Autodesk Inventor part; units mm, degrees
ref_plane "YZ Plane" through (0, 0, 0) normal (1, 0, 0) x (0, 1, 0)
ref_plane "XZ Plane" through (0, 0, 0) normal (0, 1, 0) x (-1, 0, 0)
ref_plane "XY Plane" through (0, 0, 0) normal (0, 0, 1) x (1, 0, 0)
sketch "Sketch1" plane through (0, 0, 0) normal (0, 0, 1) x (1, 0, 0)
  circle A0 centre (0, 0) radius 9.75
  dimension "d0" = 19.5
extrude "Extrusion1" add sketch "Sketch1" along normal blind 3
sketch "Sketch2" plane through (0, 0, 0) normal (0, 0, -1) x (-1, 0, 0)
  circle A0 centre (0, 0) radius 7.2
  circle A1 centre (0, 0) radius 4.7
  dimension "d3" = 14.4
  dimension "d4" = 2.5
extrude "Extrusion2" add sketch "Sketch2" along normal blind 6
fillet "Fillet1" radius 2 1 edges at (-9.75, 0, 3)
sketch "Sketch3" plane through (0, 0, 3) normal (0, 0, 1) x (1, 0, 0)
  line L0 (0.8, -4.5) -> (-0.8, -4.5)
  line L1 (-0.8, 4.5) -> (0.8, 4.5)
  line L2 (0.8, -4.5) -> (-0.8, 4.5) construction
  line L3 (-0.8, -4.5) -> (0.8, 4.5) construction
  line L4 (-3, -0.8) -> (-3, 0.8)
  line L5 (3, 0.8) -> (3, -0.8)
  circle A0 centre (0, 0) radius 4.7
  line L6 (3, -0.8) -> (-3, 0.8) construction
  line L7 (-3, -0.8) -> (3, 0.8) construction
  line L8 (3, -0.8) -> (0.8, -0.8)
  line L9 (-0.8, -4.5) -> (-0.8, -0.8)
  line L10 (0.1422, -0.8) -> (-0.1422, -0.8)
  line L11 (-0.8, -0.8) -> (-3, -0.8)
  line L12 (0.8, 0.8) -> (3, 0.8)
  line L13 (-3, 0.8) -> (-0.8, 0.8)
  line L14 (-0.1422, 0.8) -> (0.1422, 0.8)
  line L15 (-0.8, -0.2133) -> (-0.8, 0.2133)
  line L16 (-0.8, 0.8) -> (-0.8, 4.5)
  line L17 (0.8, 4.5) -> (0.8, 0.8)
  line L18 (0.8, 0.2133) -> (0.8, -0.2133)
  line L19 (0.8, -0.8) -> (0.8, -4.5)
  dimension "d8" = 9
  dimension "d9" = 6
extrude "Extrusion3" cut sketch "Sketch3" against normal blind 2 contours L0 L9 L11 L4 L13 L16 L1 L17 L12 L5 L8 L19
thread "Thread1"
chamfer "Chamfer1" distance 1 angle 45 1 edges at (7.2, 0, -6)
equation "\"d11\" = d10"
properties part number "PG9x6mm_Plug"
Here's how the part is built. I have some questions about the finished solid (model axes, mm). A direction names the side the tool comes from. Coordinates: 2 decimals unless noted, no trailing zeros. Loops run counter-clockwise (first coordinate to the right, second up) from the corner with the lowest first, then second, coordinate; pieces in that order, holes last.
1. Imagine slicing it at C-C, the plane y = 0. Please give me the cut outline in (x, z), and give its area (3 significant figures).
2. For P1, Ø1.6, axis at y = -3.5, z = 2, coming from the -X side; P2, Ø1.5, axis at y = 2.5, z = 1, coming from the -X side; P3, Ø1.6, axis at x = 2, z = 2.5, coming from the -Y side, each with a flat end and sliding along its axis, tell me the tip position at first contact or that it passes through.
3. For faces 1 (the cylindrical face through (1.02, 4.59, -2.96)), 2 (the flat face through (-2, 0.8, 2)), 3 (the flat face through (2, -2, 3)), which set-ups out of +Z, -Z, +X, -X, +Y, -Y let a thin tool reach every point of the face, with its end or its side?
4. Imagine slicing it at B-B, the plane z = -2.5. Please give me the cut outline in (x, y).
5. I need wall thicknesses on L1, parallel to Y at x = 0, z = -3.25; L2, parallel to X at y = -1.5, z = 2; L3, parallel to X at y = -2.75, z = -0.5. Which ranges of each line are inside material? Lowest first, please.
6. Imagine slicing it at D-D, the plane z = 0.25. Please give me the cut outline in (x, y), and give its area (3 significant figures).
7. If we mould it in two halves opening along X, with no side actions, what happens to faces 4 (the flat face through (1, 5, -6)), 5 (the cylindrical face through (-1.269, -9.667, 0.493)), 6 (the flat face through (0, 0, 0))? For each: pulls with the +X half, pulls with the -X half, needs draft (parallel to the pull), parting line crosses it, or undercut.
8. Imagine slicing it at A-A, the plane x = 0. Please give me the cut outline in (y, z), and give its area (3 significant figures).
Taken from the geometry:
1. outline: (-9.75, 0) - (-7.2, 0) - (-7.2, -5) - (-6.2, -6) - (-4.7, -6) - (-4.7, 0) - (4.7, 0) - (4.7, -6) - (6.2, -6) - (7.2, -5) - (7.2, 0) - (9.75, 0) - (9.75, 1) arc R2 ccw to (7.75, 3) - (3, 3) - (3, 1) - (-3, 1) - (-3, 3) - (-7.75, 3) arc R2 ccw to (-9.75, 1) - close
1. area: 73.8 mm2
2. P1: stops at x = -9.25
2. P2: stops at x = -9.59
2. P3: stops at y = -9.45
3. face 1: -Z
3. face 2: +Z
3. face 3: +Z, +X, -X, +Y, -Y
4. outline: circle Ø14.4 at (0, 0); hole circle Ø9.4 at (0, 0)
5. L1: y = -7.2 to -4.7, 4.7 to 7.2
5. L2: x = -9.36 to -0.8, 0.8 to 9.36
5. L3: x = -6.65 to -3.81, 3.81 to 6.65
6. outline: circle Ø19.5 at (0, 0)
6. area: 299 mm2
7. face 4: needs draft
7. face 5: parting line crosses it
7. face 6: undercut
8. outline: (-9.75, 0) - (-7.2, 0) - (-7.2, -5) - (-6.2, -6) - (-4.7, -6) - (-4.7, 0) - (4.7, 0) - (4.7, -6) - (6.2, -6) - (7.2, -5) - (7.2, 0) - (9.75, 0) - (9.75, 1) arc R2 ccw to (7.75, 3) - (4.5, 3) - (4.5, 1) - (-4.5, 1) - (-4.5, 3) - (-7.75, 3) arc R2 ccw to (-9.75, 1) - close
8. area: 67.8 mm2
